```python
from build123d import *

# Parameters (mm, degrees)
SKETCH1_W           = 100
SKETCH1_H           = 100
BOSS_EXTRUDE1_DEPTH = 10
SKETCH2_R           = 17.5
CUT_EXTRUDE1_DEPTH  = 3
SKETCH4_R           = 10
CUT_EXTRUDE2_DEPTH  = 7
SKETCH5_R           = 4.8
CUT_EXTRUDE3_DEPTH  = 20
SKETCH6_R           = 1.5
CUT_EXTRUDE4_DEPTH  = 5
SKETCH7_R           = 4.8
CUT_EXTRUDE5_DEPTH  = 10
SKETCH8_R           = 1.5
CUT_EXTRUDE6_DEPTH  = 5
SKETCH9_R           = 1.5
CUT_EXTRUDE7_DEPTH  = 5
SKETCH10_R          = 1.5
CUT_EXTRUDE8_DEPTH  = 5
SKETCH11_R          = 1.5
CUT_EXTRUDE9_DEPTH  = 5
CUT_EXTRUDE10_START = -5
SKETCH12_R          = 1.5
CUT_EXTRUDE10_DEPTH = 5


with BuildPart() as part:
    # Sketch1 → Boss-Extrude1 (new body)
    with BuildSketch(Plane(origin=(0, 0, 0), x_dir=(1, 0, 0), z_dir=(0, 1, 0))):
        Rectangle(SKETCH1_W, SKETCH1_H)
    extrude(amount=BOSS_EXTRUDE1_DEPTH)

    # Sketch2 → Cut-Extrude1 (cut)
    with BuildSketch(Plane(origin=(0, 10, 0), x_dir=(1, 0, 0), z_dir=(0, 1, 0))):
        with Locations(Location((-17.67766953, 17.67766953, 0), (0, 0, 270))):
            Circle(SKETCH2_R)
    extrude(amount=-CUT_EXTRUDE1_DEPTH, mode=Mode.SUBTRACT)

    # Sketch4 → Cut-Extrude2 (cut)
    with BuildSketch(Plane(origin=(0, 7, 0), x_dir=(1, 0, 0), z_dir=(0, 1, 0))):
        with Locations(Location((-17.67766953, 17.67766953, 0), (0, 0, 270))):
            Circle(SKETCH4_R)
    extrude(amount=-CUT_EXTRUDE2_DEPTH, mode=Mode.SUBTRACT)

    # Sketch5 → Cut-Extrude3 (cut)
    with BuildSketch(Plane(origin=(0, 10, 0), x_dir=(1, 0, 0), z_dir=(0, 1, 0))):
        with Locations(Location((-35.355339059, 0, 0), (0, 0, 270))):
            Circle(SKETCH5_R)
        with Locations(Location((0, 35.355339059, 0), (0, 0, 270))):
            Circle(SKETCH5_R)
    extrude(amount=-CUT_EXTRUDE3_DEPTH, mode=Mode.SUBTRACT)

    # Sketch6 → Cut-Extrude4 (cut)
    with BuildSketch(Plane(origin=(0, 10, 0), x_dir=(1, 0, 0), z_dir=(0, 1, 0))):
        with Locations(Location((-43.179859239, 17.5, 0), (0, 0, 270))):
            Circle(SKETCH6_R)
        with Locations(Location((-43.179859239, -17.5, 0), (0, 0, 90))):
            Circle(SKETCH6_R)
        with Locations(Location((17.5, 43.179859239, 0), (0, 0, 270))):
            Circle(SKETCH6_R)
        with Locations(Location((-17.5, 43.179859239, 0), (0, 0, 90))):
            Circle(SKETCH6_R)
    extrude(amount=-CUT_EXTRUDE4_DEPTH, mode=Mode.SUBTRACT)

    # Sketch7 → Cut-Extrude5 (cut)
    with BuildSketch(Plane(origin=(0, 10, 0), x_dir=(1, 0, 0), z_dir=(0, 1, 0))):
        with Locations(Location((22.32233047, -22.32233047, 0), (0, 0, 270))):
            Circle(SKETCH7_R)
    extrude(amount=-CUT_EXTRUDE5_DEPTH, mode=Mode.SUBTRACT)

    # Sketch8 → Cut-Extrude6 (cut)
    with BuildSketch(Plane(origin=(0, 10, 0), x_dir=(1, 0, 0), z_dir=(0, 1, 0))):
        with Locations(Location((40.353553391, -15.604816049, 0), (0, 0, 270))):
            Circle(SKETCH8_R)
        with Locations(Location((15.604816049, -40.353553391, 0), (0, 0, 90))):
            Circle(SKETCH8_R)
    extrude(amount=-CUT_EXTRUDE6_DEPTH, mode=Mode.SUBTRACT)

    # Sketch9 → Cut-Extrude7 (cut)
    with BuildSketch(Plane(origin=(50, 0, 0), x_dir=(0, 0, -1), z_dir=(1, 0, 0))):
        with Locations((-0.963309919, 5.096330992)):
            Circle(SKETCH9_R)
    extrude(amount=-CUT_EXTRUDE7_DEPTH, mode=Mode.SUBTRACT)

    # Sketch10 → Cut-Extrude8 (cut)
    with BuildSketch(Plane(origin=(0, 0, -50), x_dir=(-1, 0, 0), z_dir=(0, 0, -1))):
        with Locations((0, 5)):
            Circle(SKETCH10_R)
    extrude(amount=-CUT_EXTRUDE8_DEPTH, mode=Mode.SUBTRACT)

    # Sketch11 → Cut-Extrude9 (cut)
    with BuildSketch(Plane.ZY.offset(50)):
        with Locations((0, 5)):
            Circle(SKETCH11_R)
    extrude(amount=-CUT_EXTRUDE9_DEPTH, mode=Mode.SUBTRACT)

    # Sketch12 → Cut-Extrude10 (cut)
    with BuildSketch(Plane.XY.offset(50).offset(CUT_EXTRUDE10_START)):
        with Locations(Location((0, 5, 0), (0, 0, 180))):
            Circle(SKETCH12_R)
    extrude(amount=CUT_EXTRUDE10_DEPTH, mode=Mode.SUBTRACT)


solid = part.part
```
CAD build for the part. Positions are in the model's coordinates, mm. A direction names the side the tool comes from. Coordinates: 2 decimals unless noted, no trailing zeros. Order: outer loops, then holes, each group sorted by start corner. A loop starts at its lowest first (then second) coordinate and runs counter-clockwise, first axis right, second up. Notation, with made-up numbers: M -10.5,-20.75 L 23.5,-20.75 A32 ccw 23.5,9.25 Z; hole C -32.75,39 d6. An arc over 180 degrees is marked long. Write each question's results on one line, items separated by ' | '. Start each with the question number.
Q1. Pull direction X, two halves, no side cores. Call faces 1 (the cylindrical face through (-42.267, 7.535, 18.69)), 2 (the flat face through (-50, 3, 1)), 3 (the flat face through (45, 5, 1)): +X half, -X half, draft (parallel to the pull), parting line (faces both ways), or undercut.
Q2. Flat gauge pins, fed straight in: P1, Ø1.5, axis at x = -43.5, z = -18, coming from the +Y side; P2, Ø2.5, axis at y = 5.1, z = 0.96, coming from the -X side; P3, Ø0.9, axis at y = 5, z = 0, coming from the -X side; P4, Ø21, axis at x = -17.68, z = -17.68, coming from the +Y side. Where does each tip first touch, or does it go through?
Q3. Drill centre lines: probe 1 along X at (y, z) = (6.3, -17.5); probe 2 along Y at (x, z) = (0, 46); probe 3 along X at (y, z) = (5, 0). Where is each one in solid material? Low to high. Write a range as from..to.
Q4. Cut at B-B (y = 1.5). List the corners of the cut face in (x, z).
Q5. Cut at C-C (x = -24). List the corners of the cut face in (y, z), then the cut area to 3 significant figures.
Q6. Cut at A-A (z = -17.5). List the corners of the cut face in (x, y).
Q7. Which spindle directions (+Z, -Z, +X, -X, +Y, -Y) get a long thin tool onto all of the face, cutting with end or side? Do faces 4 (the flat face through (0, 5, 45)), 5 (the flat face through (0, 5, -45)), 6 (the cylindrical face through (47.535, 3.766, 0.271)), 7 (the cylindrical face through (-47.54, 5.07, -1.5)), 8 (the flat face through (-25, 7, -10)). Say none if no direction does.
Found:
1) face 1: undercut | face 2: -X half | face 3: +X half
2) P1: y = 5 | P2: x = -50 | P3: x = -45 | P4: y = 7
3) probe 1: -50..-44.68, -41.68..-27.68, -7.68..50 | probe 2: 0..3.5, 6.5..10 | probe 3: -45..-40.16, -30.56..45
4) outline: M -50,-50 L 50,-50 L 50,50 L -50,50 Z; hole C -35.36,0 d9.6; hole C -17.68,-17.68 d20; hole C 0,-35.36 d9.6; hole C 22.32,22.32 d9.6
5) outline: M 0,-50 L 10,-50 L 10,-34 L 7,-34 L 7,-25.43 L 0,-25.43 Z; M 0,-9.93 L 7,-9.93 L 7,-1.36 L 10,-1.36 L 10,50 L 0,50 Z | area: 794 mm²
6) outline: M -50,0 L -27.68,0 L -27.68,7 L -35.18,7 L -35.18,10 L -41.68,10 L -41.68,5 L -44.68,5 L -44.68,10 L -50,10 Z; M -7.68,0 L 50,0 L 50,10 L -0.18,10 L -0.18,7 L -7.68,7 Z
7) face 4: +Z | face 5: -Z | face 6: +X | face 7: -X | face 8: +Y
